from build123d import *

# Parameters (mm, degrees)
SKETCH1_W           = 6.35
SKETCH1_H           = 734.741844671
BOSS_EXTRUDE1_DEPTH = 107.95
SKETCH2_W           = 6.35
SKETCH2_H           = 734.741844671
BOSS_EXTRUDE2_DEPTH = 120.65


with BuildPart() as part:
    # Sketch1 → Boss-Extrude1 (new body)
    with BuildSketch(Plane.XY):
        with Locations((194.071875, 89.829077665)):
            Rectangle(SKETCH1_W, SKETCH1_H)
    extrude(amount=BOSS_EXTRUDE1_DEPTH)

    # Sketch2 → Boss-Extrude2 (add)
    with BuildSketch(Plane.ZY.offset(-190.896875)):
        with Locations((104.775, 89.829077665)):
            Rectangle(SKETCH2_W, SKETCH2_H)
    extrude(amount=BOSS_EXTRUDE2_DEPTH)


solid = part.part
Geometry: final body of the model. Coordinates: model frame, mm. A direction names the side the tool comes from. Give positions to 0.01 mm unless a question says otherwise; leave off trailing zeros. Write each loop counter-clockwise with the first axis right and the second up, starting at its lowest first coordinate (ties: lowest second). Pieces come first, ordered by that corner, then holes. Notation, with made-up numbers: (34, -7.75) -> (53, -7.75) arc R12 ccw to (53, 0.25) -> close; hole circle Ø8 at (35, 81). An arc over 180 degrees is marked (long way). Answer in a Markdown table with one row per item.
(1) Ray query, line 1 along Z through (x, y) = (103.5, -192); line 2 along X through (y, z) = (-44.5, 35.5). Return the intervals inside material, ascending. Write a range as [from, to].
Answers below:
| item | result |
|---|---|
| line 1 | [101.6, 107.95] |
| line 2 | [190.9, 197.25] |
(2) Section query B-B on x = 167. Return loops of the section in (y, z).
Answers below:
| item | result |
|---|---|
| outline | (-277.54, 101.6) -> (457.2, 101.6) -> (457.2, 107.95) -> (-277.54, 107.95) -> close |
(3) Section query C-C on z = 88. Return loops of the section in (x, y), then the cut area to 3 significant figures.
Answers below:
| item | result |
|---|---|
| outline | (190.9, -277.54) -> (197.25, -277.54) -> (197.25, 457.2) -> (190.9, 457.2) -> close |
| area | 4,670 mm^2 |
(4) Pin query (flat end, axial travel): pin 1 (8 mm diameter, centred on y = 14.5, z = 17.5, fed in from -X). Return the tip coordinate at first contact, or that it passes through.
Answers below:
| item | result |
|---|---|
| pin 1 | x = 190.9 |
(5) Set-up query: faces 1 (the flat face through (190.897, 85, 50)), 2 (the flat face through (153, 457.2, 102)). Return all of +Z, -Z, +X, -X, +Y, -Y with unobstructed straight access to the full face (end or side cutting, diameter ignored); none if empty.
Answers below:
| item | result |
|---|---|
| face 1 | -Z, -X, +Y, -Y |
| face 2 | +Z, -Z, +X, -X, +Y |
(6) Section query A-A on y = 235.5. Return loops of the section in (x, z), then the cut area to 3 significant figures.
Answers below:
| item | result |
|---|---|
| outline | (70.25, 101.6) -> (190.9, 101.6) -> (190.9, 0) -> (197.25, 0) -> (197.25, 107.95) -> (70.25, 107.95) -> close |
| area | 1,450 mm^2 |
